Geometry: final body of the model. Coordinates: model frame, mm. Face numbers are marked on the shaded views. A direction names the side the tool comes from. Give positions to 0.01 mm unless a question says otherwise; leave off trailing zeros. Order: outer loops, then holes, each group sorted by start corner. A loop starts at its lowest first (then second) coordinate and runs counter-clockwise, first axis right, second up. Notation, with made-up numbers: (48.25, 72.5) -> (70.25, 72.5) arc R34 ccw to (70.25, 107.5) -> close; hole circle Ø4 at (70.5, 70). An arc over 180 degrees is marked (long way). Write item = value, one per line.
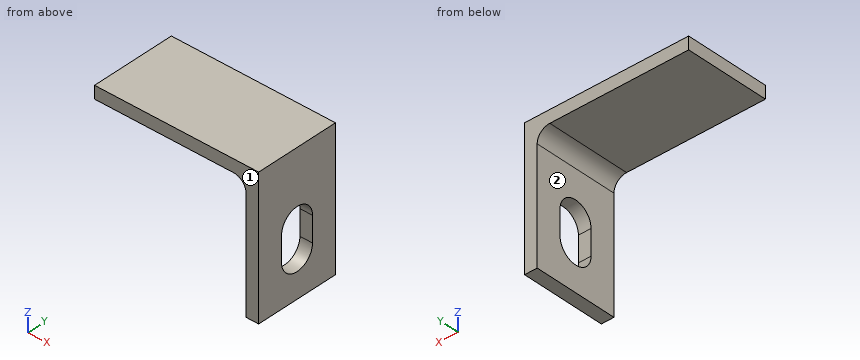
Solid Edge part; units mm, degrees
sketch "Sketch1" plane through (191.4483, 0, 0) normal (1, 0, 0) x (0, 1, 0)
  line L0 (43, 6.225) -> (43, -15.7)
  line L1 (43, -15.7) -> (56.4, -15.7)
  line L2 (56.4, -15.7) -> (56.4, 6.225)
  line L3 (43, 6.225) -> (56.4, 6.225)
  arc A0 (47, -5) -> (52.4, -5) centre (49.7, -5) cw
  line L4 (52.4, -5) -> (52.4, -9)
  arc A1 (52.4, -9) -> (47, -9) centre (49.7, -9) cw
  line L5 (47, -5) -> (47, -9)
extrude "ExtrudedProtrusion_1" add sketch "Sketch1" against normal blind 2
sketch "Sketch2" plane through (189.4483, 49.7, -4.7375) normal (-1, 0, 0) x (0, -1, 0)
  line L0 (6.7, 8.9625) -> (-6.7, 8.9625)
  line L1 (-6.7, 8.9625) -> (-6.7, 10.9625)
  line L2 (-6.7, 10.9625) -> (6.7, 10.9625)
  line L3 (6.7, 10.9625) -> (6.7, 8.9625)
extrude "ExtrudedProtrusion_2" add sketch "Sketch2" along normal blind 30
fillet "Round_1" radius 2 1 edges at (189.4483, 49.7, 4.225)
sketch "Sketch3" plane through (174.4483, 49.7, 6.225) normal (0, 0, 1) x (1, 0, 0)
  line L0 (-15, 6.7) -> (-9, 6.7)
  line L1 (-9, 6.7) -> (-9, -8.8596)
  dimension "D1" = 15
extrude "Cutout1" cut sketch "Sketch3" against normal through all material side at (162.4483, 56.35, 6.225)
properties material "ABS Plastic, medium impact"
1) Section query B-B (z = -4.5). Output: boundary loops of the cut face in (x, y).
Check sheet entries:
outline = (189.45, 43) -> (191.45, 43) -> (191.45, 47.05) -> (189.45, 47.05) -> close; (189.45, 52.35) -> (191.45, 52.35) -> (191.45, 56.4) -> (189.45, 56.4) -> close
2) Section query D-D (y = 55). Output: boundary loops of the cut face in (x, z) (3 decimals), plus the area to 3 significant figures.
Check sheet entries:
outline = (165.448, 4.225) -> (187.448, 4.225) arc R2 cw to (189.448, 2.225) -> (189.448, -15.7) -> (191.448, -15.7) -> (191.448, 6.225) -> (165.448, 6.225) -> close
area = 92.7 mm²
3) Section query A-A (y = 49.7). Output: boundary loops of the cut face in (x, z) (3 decimals).
Check sheet entries:
outline = (165.448, 4.225) -> (187.448, 4.225) arc R2 cw to (189.448, 2.225) -> (189.448, -2.3) -> (191.448, -2.3) -> (191.448, 6.225) -> (165.448, 6.225) -> close; (189.448, -15.7) -> (191.448, -15.7) -> (191.448, -11.7) -> (189.448, -11.7) -> close
4) First-contact query: P1, Ø1.5, axis at y = 54.5, z = 2.5, coming from the -X side; P2, Ø1, axis at y = 47, z = -11, coming from the -X side; P3, Ø8, axis at x = 171.5, y = 47.5, coming from the -Z side (3 decimals). Flat tips, straight axial feed; report the tip coordinate or a pass-through.
Check sheet entries:
P1 = 189.17
P2 = 189.45
P3 = 4.225
5) Reachability of the marked faces 1 and 2 from +Z, -Z, +X, -X, +Y, -Y: full face, straight path, thin tool, end or side. Return the list, or none.
Check sheet entries:
face_1 = +Z, -Z, +X, -X, -Y
face_2 = -Z, -X, +Y, -Y
6) Line query: line 1 (X direction, y = 44.75, z = -13.5); line 2 (Z direction, x = 177.25, y = 44.25) (3 decimals); line 3 (X direction, y = 55, z = 4). Output: solid intervals per line, ascending. Write a range as from..to.
Check sheet entries:
line_1 = 189.45..191.45
line_2 = 4.225..6.225
line_3 = 188.37..191.45
7) Section query C-C (x = 185.5). Output: boundary loops of the cut face in (y, z) (3 decimals).
Check sheet entries:
outline = (43, 4.225) -> (56.4, 4.225) -> (56.4, 6.225) -> (43, 6.225) -> close
